The model under review builds one solid part; all positions refer to its coordinate system, in mm. Face numbers are marked on the shaded views. A direction names the side the tool comes from. Round coordinates to 2 decimals unless told otherwise and drop trailing zeros. Loops run counter-clockwise (first coordinate to the right, second up) from the corner with the lowest first, then second, coordinate; pieces in that order, holes last. Notation, with made-up numbers: (39.25, 42.5) - (87.25, 42.5) arc R24 cw to (87.25, 62.5) - close; hole circle Ø8 at (-7.5, 42). An arc over 180 degrees is marked (long way). Answer as CSV lines item,"result".
from build123d import *

# Parameters (mm, degrees)
SKETCH1_W             = 2032
SKETCH1_H             = 152.4
BOSS_EXTRUDE1_DEPTH   = 50.8
BOSS_EXTRUDE1_2_DEPTH = 50.8
BOSS_EXTRUDE1_3_DEPTH = 50.8
BOSS_EXTRUDE1_4_DEPTH = 50.8
BOSS_EXTRUDE1_5_DEPTH = 50.8
SKETCH2_W             = 1930.4
SKETCH2_H             = 685.8
SKETCH2_W_2           = 1828.8
SKETCH2_H_2           = 584.2
BOSS_EXTRUDE2_DEPTH   = 203.2


with BuildPart() as part:
    # Sketch1 → Boss-Extrude1 (new body)
    with BuildSketch(Plane(origin=(0, 0, 0), x_dir=(1, 0, 0), z_dir=(0, 1, 0))):
        Rectangle(SKETCH1_W, SKETCH1_H)
    extrude(amount=BOSS_EXTRUDE1_DEPTH)



with BuildPart() as body_2:
    # Sketch1 → Boss-Extrude1 2 (new body)
    with BuildSketch(Plane(origin=(0, 0, 0), x_dir=(1, 0, 0), z_dir=(0, 1, 0))):
        with Locations((0, 158.75)):
            Rectangle(SKETCH1_W, SKETCH1_H)
    extrude(amount=BOSS_EXTRUDE1_2_DEPTH)


with BuildPart() as body_3:
    # Sketch1 → Boss-Extrude1 3 (new body)
    with BuildSketch(Plane(origin=(0, 0, 0), x_dir=(1, 0, 0), z_dir=(0, 1, 0))):
        with Locations((0, 317.5)):
            Rectangle(SKETCH1_W, SKETCH1_H)
    extrude(amount=BOSS_EXTRUDE1_3_DEPTH)


with BuildPart() as body_4:
    # Sketch1 → Boss-Extrude1 4 (new body)
    with BuildSketch(Plane(origin=(0, 0, 0), x_dir=(1, 0, 0), z_dir=(0, 1, 0))):
        with Locations((0, -158.75)):
            Rectangle(SKETCH1_W, SKETCH1_H)
    extrude(amount=BOSS_EXTRUDE1_4_DEPTH)


with BuildPart() as body_5:
    # Sketch1 → Boss-Extrude1 5 (new body)
    with BuildSketch(Plane(origin=(0, 0, 0), x_dir=(1, 0, 0), z_dir=(0, 1, 0))):
        with Locations((0, -317.5)):
            Rectangle(SKETCH1_W, SKETCH1_H)
    extrude(amount=BOSS_EXTRUDE1_5_DEPTH)


with BuildPart() as part_1:
    add(part.part)

    add(body_2.part)  # Boss-Extrude2 merges body 2

    add(body_3.part)  # Boss-Extrude2 merges body 3

    add(body_4.part)  # Boss-Extrude2 merges body 4

    add(body_5.part)  # Boss-Extrude2 merges body 5
    # Sketch2 → Boss-Extrude2 (add)
    with BuildSketch(Plane(origin=(0, 0, 0), x_dir=(-1, 0, 0), z_dir=(0, -1, 0))):
        Rectangle(SKETCH2_W, SKETCH2_H)
        Rectangle(SKETCH2_W_2, SKETCH2_H_2, mode=Mode.SUBTRACT)
    extrude(amount=BOSS_EXTRUDE2_DEPTH)


solid = part_1.part
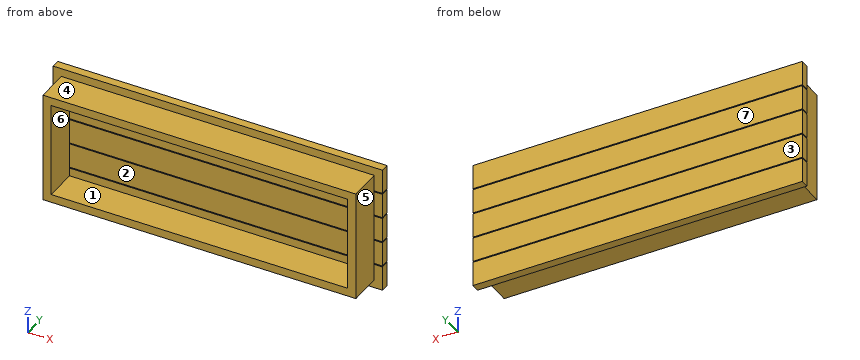
1. Wall thickness on probe 1 along Z at (x, y) = (488.5, -4); probe 2 along X at (y, z) = (-171.5, 135.5); probe 3 along Y at (x, z) = (395, 104): over which ranges is each line inside the solid? List them lowest first.
Numbers:
probe 1,"z = -342.9 to -292.1, 292.1 to 342.9"
probe 2,"x = -965.2 to -914.4, 914.4 to 965.2"
probe 3,"y = 0 to 50.8"
2. Take a section at C-C (z = 165). State the section outline as (x, y) points.
Numbers:
outline,"(-1016, 0) - (-965.2, 0) - (-965.2, -203.2) - (-914.4, -203.2) - (-914.4, 0) - (914.4, 0) - (914.4, -203.2) - (965.2, -203.2) - (965.2, 0) - (1016, 0) - (1016, 50.8) - (-1016, 50.8) - close"
3. Take a section at B-B (x = -464.5). State the section outline as (y, z) points.
Numbers:
outline,"(-203.2, -342.9) - (0, -342.9) - (0, -393.7) - (50.8, -393.7) - (50.8, -241.3) - (0, -241.3) - (0, -292.1) - (-203.2, -292.1) - close; (-203.2, 292.1) - (0, 292.1) - (0, 241.3) - (50.8, 241.3) - (50.8, 393.7) - (0, 393.7) - (0, 342.9) - (-203.2, 342.9) - close; (0, -234.95) - (50.8, -234.95) - (50.8, -82.55) - (0, -82.55) - close; (0, -76.2) - (50.8, -76.2) - (50.8, 76.2) - (0, 76.2) - close; (0, 82.55) - (50.8, 82.55) - (50.8, 234.95) - (0, 234.95) - close"
4. Clearance check with flat-ended pins moving along their axes: pin 1 (5 mm diameter, centred on y = -51, z = -105.5, fed in from +X); pin 2 (12 mm diameter, centred on x = -90, z = -257, fed in from -Y); pin 3 (1.9 mm diameter, centred on x = 951.5, z = 237, fed in from +Y). State where each tip first meets the part, or that it passes through.
Numbers:
pin 1,"stops at x = 965.2"
pin 2,"stops at y = 0"
pin 3,"stops at y = 0"
5. Take a section at A-A (y = -88.5). State the section outline as (x, z) points, plus the area to 3 significant figures.
Numbers:
outline,"(-965.2, -342.9) - (965.2, -342.9) - (965.2, 342.9) - (-965.2, 342.9) - close; hole (-914.4, -292.1) - (914.4, -292.1) - (914.4, 292.1) - (-914.4, 292.1) - close"
area,"255,000 mm²"
6. Draft analysis for pull direction Y (two halves, no side actions). For the marked faces 1, 2 and 3, state which applies: +Y half, -Y half, draft (parallel to the pull), parting line (faces both ways), or undercut.
Numbers:
face 1,"draft"
face 2,"-Y half"
face 3,"+Y half"
7. Take a section at D-D (y = 23.5). State the section outline as (x, z) points.
Numbers:
outline,"(-1016, -393.7) - (1016, -393.7) - (1016, -241.3) - (-1016, -241.3) - close; (-1016, -234.95) - (1016, -234.95) - (1016, -82.55) - (-1016, -82.55) - close; (-1016, -76.2) - (1016, -76.2) - (1016, 76.2) - (-1016, 76.2) - close; (-1016, 82.55) - (1016, 82.55) - (1016, 234.95) - (-1016, 234.95) - close; (-1016, 241.3) - (1016, 241.3) - (1016, 393.7) - (-1016, 393.7) - close"
8. Tool access review of the marked faces 4, 5, 6 and 7: name each direction out of +Z, -Z, +X, -X, +Y, -Y from which nothing blocks a thin tool from reaching the whole face with its end or side.
Numbers:
face 4,"+Z, +X, -X, -Y"
face 5,"+Z, -Z, +X, -Y"
face 6,"-Y"
face 7,"+Z, -Z, +X, -X, +Y"
